Can you work these out from the drawing? Everything is in mm from the part's minimum corner. A direction names the side the tool comes from. Coordinates: 2 decimals unless noted, no trailing zeros. Loops run counter-clockwise (first coordinate to the right, second up) from the corner with the lowest first, then second, coordinate; pieces in that order, holes last. Notation, with made-up numbers: (1.5, 4.25) -> (31.5, 4.25) arc R22 ccw to (31.5, 16.25) -> close; hole circle Ø1 at (83.5, 1). An arc over 180 degrees is marked (long way). Put each result on its own line as item: value. Start each with the question number.
Item 1: Please list where these lines run through material, in increasing order: L1, parallel to Y at x = 8, z = 170.5; L2, parallel to Z at x = 9, y = 31.5; L3, parallel to X at y = 80.5, z = 85. Write a range as from..to.
Item 2: If we section it at C-C on y = 42.5: Please give me the cut outline in (x, z), plus the area to 3 significant figures.
Item 3: Will these pins go through, and if not, where does the flat tip stop? P1, Ø4, axis at x = 32, y = 25, coming from the +Z side; P2, Ø9.5, axis at y = 62, z = 113, coming from the +X side; P3, Ø11, axis at x = 22, z = 41.5, coming from the -Y side; P4, Ø7.5, axis at x = 18.5, z = 168, coming from the +Y side.
Item 4: If we section it at D-D on x = 13: Please give me the cut outline in (y, z).
Item 5: For the marked faces 1, 2, 3 and 4, which set-ups out of +Z, -Z, +X, -X, +Y, -Y let a thin tool reach every point of the face, with its end or its side?
Item 6: If we section it at B-B on z = 20.5: Please give me the cut outline in (x, y).
Item 7: If we section it at A-A on y = 62: Please give me the cut outline in (x, z), plus the area to 3 significant figures.
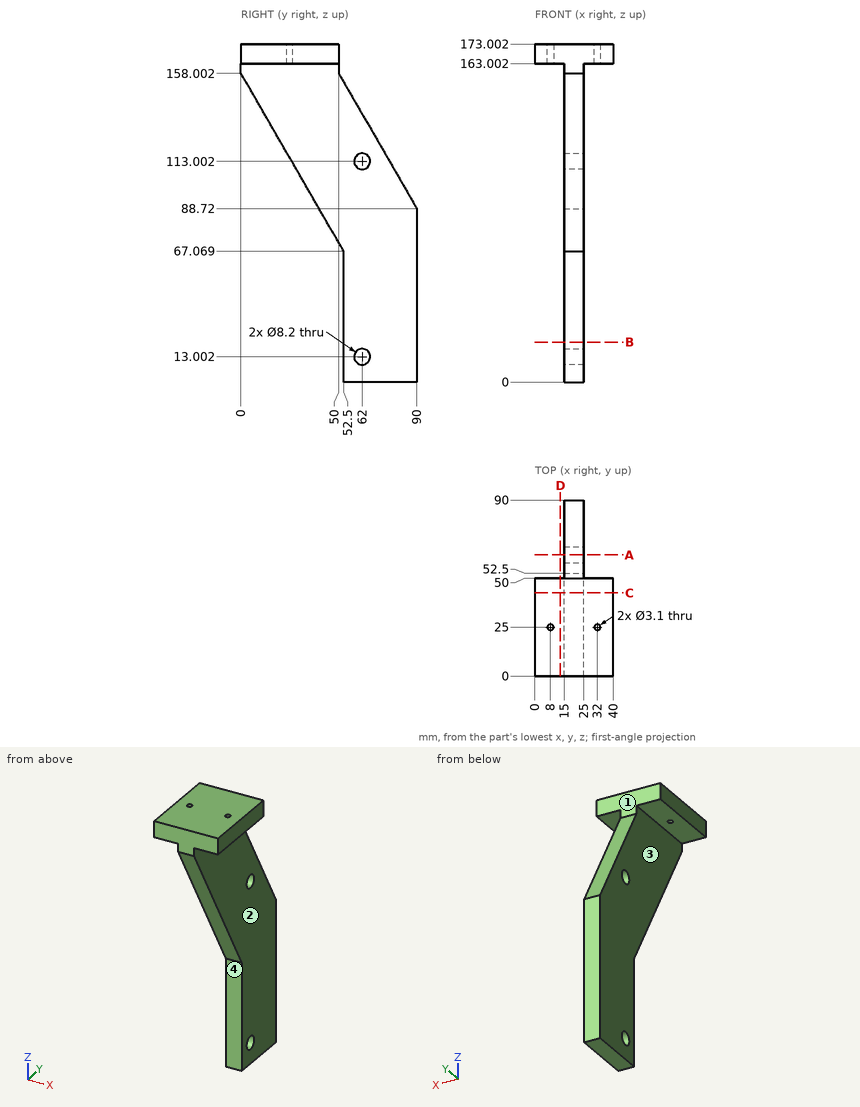
Solutions:
1. L1: 0..23.45, 26.55..50
1. L2: 163..173
1. L3: 15..25
2. outline: (0, 163) -> (15, 163) -> (15, 84.39) -> (25, 84.39) -> (25, 163) -> (40, 163) -> (40, 173) -> (0, 173) -> close
2. area: 1,190 mm^2
3. P1: z = 173
3. P2: x = 25
3. P3: y = 52.5
3. P4: y = 50
4. outline: (0, 163) -> (50, 163) -> (50, 173) -> (0, 173) -> close
5. face 1: +Z, +X, -X, +Y
5. face 2: -Z, +X, +Y, -Y
5. face 3: -Z, -X, +Y, -Y
5. face 4: -Z, +X, -X, -Y
6. outline: (15, 52.5) -> (25, 52.5) -> (25, 90) -> (15, 90) -> close
7. outline: (15, 0) -> (25, 0) -> (25, 8.9) -> (15, 8.9) -> close; (15, 17.1) -> (25, 17.1) -> (25, 108.9) -> (15, 108.9) -> close; (15, 117.1) -> (25, 117.1) -> (25, 137.22) -> (15, 137.22) -> close
7. area: 1,210 mm^2
